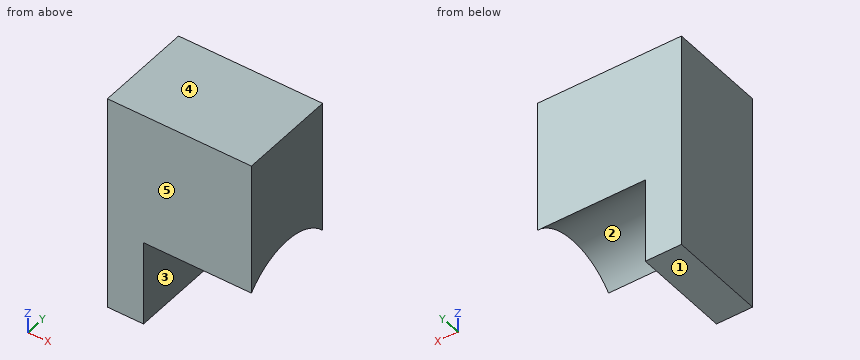
from build123d import *

# Parameters (mm, degrees)
F1_DEPTH   = 23
F1_FACE1_W = 23
F1_FACE1_H = 51.7166927457
F3_DEPTH   = 25.4


with BuildPart() as f1:
    # F0 (on Front) → F1 (new body)
    with BuildSketch(Plane.XZ):
        Polygon((41.91, 51.7166927457), (41.91, 51.36642), (41.91, 0), (75.8052021265, 0), (75.8052021265, 51.7166927457), align=None)
    extrude(amount=-F1_DEPTH)

    # F2 (on face) + F1_face1 (on face) → F3 (cut)
    with BuildSketch(Plane.YZ.offset(75.8052021265)):
        with BuildLine():
            Line((0, 0), (23, 0))
            ThreePointArc((23, 0), (11.5, 25.3947172526), (0, 0))
        make_face()
    with BuildSketch(Plane(origin=(41.91, 11.5, 25.8583463728), x_dir=(0, -1, 0), z_dir=(-1, 0, 0))):
        Rectangle(F1_FACE1_W, F1_FACE1_H)
    extrude(amount=-F3_DEPTH, dir=(1, 0, 0), mode=Mode.SUBTRACT)


solid = f1.part
Could you check a few things on this model? Use its own coordinates, in mm. Face numbers are marked on the shaded views. A direction names the side the tool comes from. Give positions to 0.01 mm unless a question says otherwise; leave off trailing zeros. Order: outer loops, then holes, each group sorted by start corner. A loop starts at its lowest first (then second) coordinate and runs counter-clockwise, first axis right, second up. Notation, with made-up numbers: (-2, 53) - (22, 53) arc R15 ccw to (22, 67) - close; hole circle Ø7 at (39, 9). An arc over 180 degrees is marked (long way). One line per question, with ' | ' between items. Start each with the question number.
Item 1: I'm going to push a flat-ended pin straight in: pin 1 Ø8 at (x, y) = (71, 10.5) entering from -Z. Where does the tip first touch, or does it pass through?
Item 2: For the marked faces 1 and 2, which set-ups out of +Z, -Z, +X, -X, +Y, -Y let a thin tool reach every point of the face, with its end or its side?
Item 3: I want a section at B-B on z = 19. Write out the boundary of the cut face in (x, y), then the cut area to 3 significant figures.
Item 4: Thinking about a two-plate mould opening in Y: for the marked faces 3, 4 and 5, which applies, pulls with the +Y half, pulls with the -Y half, needs draft (parallel to the pull), parting line crosses it, or undercut?
Item 5: I want a section at C-C on y = 2.25. Write out the boundary of the cut face in (x, z), then the cut area to 3 significant figures.
Item 6: I want a section at D-D on y = 11.5. Write out the boundary of the cut face in (x, z).
Item 7: I want a section at A-A on x = 60. Write out the boundary of the cut face in (y, z), then the cut area to 3 significant figures.
Item 8: I need wall thicknesses on probe 1 along X at (y, z) = (16, 11); probe 2 along Z at (x, y) = (61, 2); probe 3 along Z at (x, y) = (55, 2.5). Which ranges of each line are inside material? Lowest first, please. Write a range as [from, to].
Verdict:
1) pin 1: z = 24.55
2) face 1: -Z, +X, -X, +Y, -Y | face 2: -Z, +X
3) outline: (41.91, 0) - (50.41, 0) - (50.41, 23) - (41.91, 23) - close | area: 195 mm^2
4) face 3: undercut | face 4: needs draft | face 5: pulls with the -Y half
5) outline: (41.91, 0) - (50.41, 0) - (50.41, 22.28) - (75.81, 22.28) - (75.81, 51.72) - (41.91, 51.72) - close | area: 1,190 mm^2
6) outline: (41.91, 0) - (50.41, 0) - (50.41, 25.39) - (75.81, 25.39) - (75.81, 51.72) - (41.91, 51.72) - close
7) outline: (0, 20.19) arc R15.3 cw to (23, 20.19) - (23, 51.72) - (0, 51.72) - close | area: 642 mm^2
8) probe 1: [41.91, 50.41] | probe 2: [22.09, 51.72] | probe 3: [22.47, 51.72]
